The listing builds one solid part. Answer for the finished solid, in the listing's coordinates (mm). A direction names the side the tool comes from. Round coordinates to 2 decimals unless told otherwise and drop trailing zeros. Write each loop counter-clockwise with the first axis right and the second up, starting at its lowest first coordinate (ties: lowest second). Pieces come first, ordered by that corner, then holes. Notation, with made-up numbers: (3.25, -5.5) - (39.25, -5.5) arc R20 cw to (39.25, -0.5) - close; hole circle Ø8 at (17, 39). An arc over 180 degrees is marked (long way). Answer as CSV lines item,"result". Start each with the question number.
Item 1: A cutting plane is placed at B-B on y = -11. State how many separate pieces and enclosed holes the cut face has, and give its area (3 significant figures).
Item 2: A cutting plane is placed at C-C on z = -17.5. Determine the outline of the cut face in (x, y), and give its area (3 significant figures).
Item 3: Which of the six approach directions +Z, -Z, +X, -X, +Y, -Y give full straight-line access (tool end or side, diameter ignored) to faces 1 (the cylindrical face through (19.076, 4.93, 6.007)), 2 (the cylindrical face through (-72.938, 7.078, 11.143))?
Item 4: For a pull along Z with two mould halves and no side action, classify faces 3 (the cylindrical face through (-110.98, 4.93, 0.88)), 4 (the cylindrical face through (-113.48, 4.93, 0.99)), 5 (the flat face through (-20.1, 10, 1.6)) as pulls with the +Z half, pulls with the -Z half, needs draft (parallel to the pull), parting line crosses it, or undercut.
Item 5: Straight lines are drawn through the part: line 1 along X through (y, z) = (8, 0); line 2 along Z through (x, y) = (-91, 6.75); line 3 along X through (y, z) = (5, -11.5). For each, find the intervals that lie inside material, in ascending order. Write a range as [from, to].
Item 6: A cutting plane is placed at A-A on z = 0. Determine the outline of the cut face in (x, y), and give its area (3 significant figures).
Item 7: Flat-ended cylindrical pins translate along their axes: pin 1 (12 mm diameter, centred on y = -20.5, z = 2.5, fed in from +X); pin 2 (5 mm diameter, centred on y = -48.5, z = 3, fed in from -X); pin 3 (1 mm diameter, centred on x = -79.5, z = 15, fed in from -Y). Find the tip coordinate at first contact, or state that the pin passes through.
Autodesk Inventor part; units mm, degrees
ref_plane "Work Plane2" through (-91, 10, 0) normal (0.8290376, 0, 0.5591929) x (0, 1, 0)
ref_plane "XZ Plane" through (0, 0, 0) normal (0, 1, 0) x (-1, 0, 0)
ref_plane "XY Plane" through (0, 0, 0) normal (0, 0, 1) x (1, 0, 0)
sketch "Sketch1" plane through (0, 0, 0) normal (0, 1, 0) x (-1, 0, 0)
  circle A0 centre (0, 0) radius 20
  circle A1 centre (0, 0) radius 22.5
  dimension "d0" = 40
  dimension "d1" = 45
sketch "Sketch2" plane through (0, 0, 0) normal (0, 0, 1) x (1, 0, 0)
  arc A0 (-91, 0) -> (0, 0) centre (-45.5, 0) ccw
  dimension "d34" = 91
sweep "Sweep2" add profiles "Sketch1" path "Sketch2"
sketch "Sketch3" plane through (-91, 0, 0) normal (0, 1, 0) x (1, 0, 0)
  circle A0 centre (0, 0) radius 20
  circle A1 centre (0, 0) radius 22.5
  circle A2 centre (91, 0) radius 20
  circle A3 centre (91, 0) radius 22.5
extrude "Extrusion1" add sketch "Sketch3" along normal blind 10
ref_plane "Work Plane1" through (0, 0, 0) normal (0.8290376, 0, 0.5591929) x (0, 1, 0)
sketch "Sketch4" plane through (0, 0, 0) normal (0.8290376, 0, 0.5591929) x (0, 1, 0)
  line L0 (10, -22.5) -> (10, 22.5)
  line L1 (0, 22.5) -> (0, -22.5)
  point P0 (0, 0)
  point P1 (5, 0)
  dimension "d14" = 5
  dimension "d15" = 22.5
  dimension "d16" = 22.5
hole "Hole1" at (0, 5, 0) direction (-0.8290376, 0, -0.5591929) diameter 4.5 end up to surface
sketch "Sketch5" plane through (-91, 10, 0) normal (0, 1, 0) x (1, 0, 0)
  point P0 (91, 0)
  point P1 (0, 0)
  point P2 (0, 0)
ref_plane "Work Plane2" through (-91, 10, 0) normal (0.8290376, 0, 0.5591929) x (0, 1, 0)
sketch "Sketch6" plane through (-91, 10, 0) normal (0.8290376, 0, 0.5591929) x (0, 1, 0)
  line L0 (0, -22.5) -> (0, 22.5)
  line L1 (-10, -22.5) -> (-10, 22.5)
  line L2 (-10, -22.5) -> (0, -22.5)
  line L3 (-10, 22.5) -> (0, 22.5)
  point P0 (-10, -50.8866)
  point P1 (-5, 0)
  dimension "d24" = 5
  dimension "d25" = 22.5
  dimension "d26" = 22.5
hole "Hole2" at (-91, 5, 0) direction (0.8290376, 0, 0.5591929) diameter 4.5 end up to surface
properties part number "Pancake_Flexi Pipe Flipped" material "PMMA Plastic"
Geometry says:
1,separate pieces,"2"
1,enclosed holes,"2"
1,area,"699 mm^2"
2,outline,"(-105.14, 0) arc R59.64 ccw to (14.14, 0) - (14.14, 10) - (9.68, 10) - (9.68, 0) arc R55.18 cw to (-100.68, 0) - (-100.68, 10) - (-105.14, 10) - close; (-81.32, 0) arc R35.82 ccw to (-9.68, 0) - (-9.68, 10) - (-14.14, 10) - (-14.14, 0) arc R31.36 cw to (-76.86, 0) - (-76.86, 10) - (-81.32, 10) - close"
2,area,"1,450 mm^2"
3,face 1,"+Y"
3,face 2,"none"
4,face 3,"undercut"
4,face 4,"parting line crosses it"
4,face 5,"needs draft"
5,line 1,"x = [-113.5, -111], [-71, -68.5], [-22.5, -20], [20, 22.5]"
5,line 2,"z = [-22.5, -20], [20, 22.5]"
5,line 3,"x = [-110.34, -107.36], [-74.64, -71.66], [16.36, 19.34]"
6,outline,"(-113.5, 0) arc R68 ccw to (22.5, 0) - (22.5, 10) - (20, 10) - (20, 0) arc R65.5 cw to (-111, 0) - (-111, 10) - (-113.5, 10) - close; (-71, 0) arc R25.5 ccw to (-20, 0) - (-20, 10) - (-22.5, 10) - (-22.5, 0) arc R23 cw to (-68.5, 0) - (-68.5, 10) - (-71, 10) - close"
6,area,"815 mm^2"
7,pin 1,"stops at x = 20.87"
7,pin 2,"stops at x = -95.35"
7,pin 3,"stops at y = -52.78"
